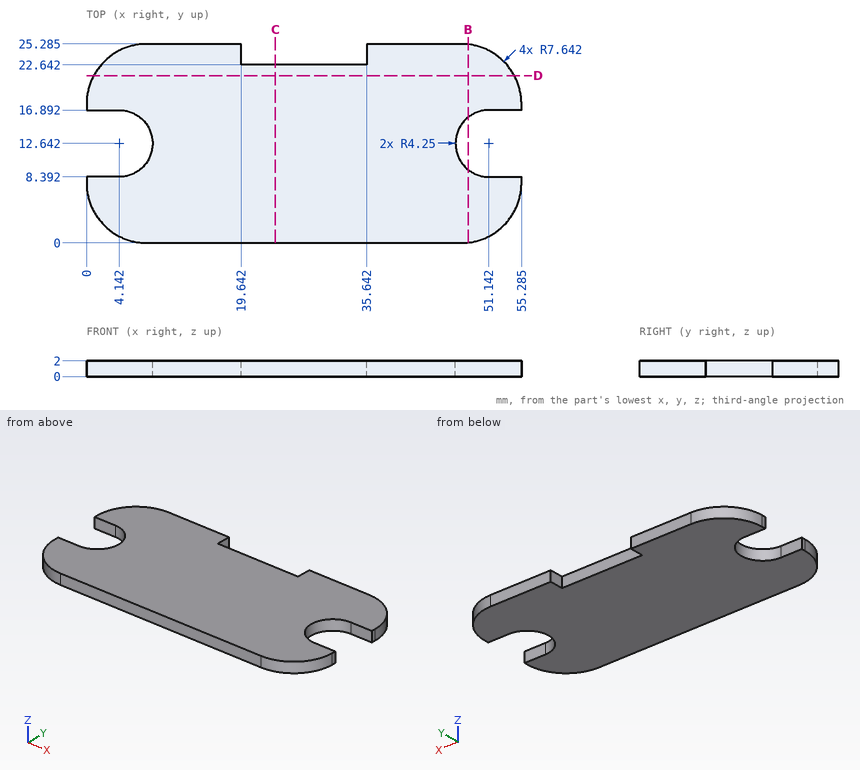
Verification items for this drawing (mm, ordinates from the low corner). Round coordinates to 2 decimals unless told otherwise and drop trailing zeros. Order: outer loops, then holes, each group sorted by start corner. A loop starts at its lowest first (then second) coordinate and runs counter-clockwise, first axis right, second up.
1) Cross-section at D-D, the plane y = 21.25. Record the cut outline in (x, z) (1 decimal).
Geometry says:
outline: (0.9, 0) - (54.4, 0) - (54.4, 2) - (0.9, 2) - close
2) Material ranges on line 1 (Y direction, x = 23, z = 0.2); line 2 (Y direction, x = 48, z = 0.35) (1 decimal); line 3 (Y direction, x = 8, z = 1.05) (1 decimal), recorded low to high.
Geometry says:
line 1: y = 0 to 22.64
line 2: y = 0 to 9.8, 15.5 to 25.3
line 3: y = 0 to 10.9, 14.4 to 25.3
3) Cross-section at B-B, the plane x = 48.5. Record the cut outline in (y, z).
Geometry says:
outline: (0.05, 0) - (9.31, 0) - (9.31, 2) - (0.05, 2) - close; (15.97, 0) - (25.24, 0) - (25.24, 2) - (15.97, 2) - close
4) Cross-section at C-C, the plane x = 24. Record the cut outline in (y, z).
Geometry says:
outline: (0, 0) - (22.64, 0) - (22.64, 2) - (0, 2) - close
5) Depth check by flat-ended pin: pin 1 (0.6 mm diameter, centred on y = 24.5, z = 1, fed in from +X) (1 decimal); pin 2 (1 mm diameter, centred on x = 53.5, z = 0.5, fed in from -Y); pin 3 (1 mm diameter, centred on x = 3, z = 0.5, fed in from +Y) (1 decimal). Enter the tip coordinate at first touch or a pass-through.
Geometry says:
pin 1: stops at x = 51.6
pin 2: stops at y = 2.19
pin 3: stops at y = 24.1
